CAD build for the part. Positions are in the model's coordinates, mm. A direction names the side the tool comes from. Give positions to 0.01 mm unless a question says otherwise; leave off trailing zeros. Write each loop counter-clockwise with the first axis right and the second up, starting at its lowest first coordinate (ties: lowest second). Pieces come first, ordered by that corner, then holes. Notation, with made-up numbers: (71.5, 32.5) - (114.5, 32.5) arc R10 cw to (114.5, 41.5) - close; hole circle Ø6 at (14, -8). An arc over 180 degrees is marked (long way). Answer as a JSON object with one key per item and string values.
from build123d import *

# Parameters (mm, degrees)
MAIN_CASE_OUTLINE_DEPTH      = 6.02
MAIN_CASE_OUTLINE_DEPTH_BACK = 6.185
SKETCH2_W                    = 78.2
SKETCH2_H                    = 5
GASKET_CUTOUTS_DEPTH         = 4
MAKE_START                   = -9.185
MAKE_ROOM_FOR_BATTERY_DEPTH  = 3
SOLIDIFY_BOTTOM_DEPTH        = 2
MOVE_FACE2_BY                = 15


# Read off the part's stored shape, not the designer's step: Make Room for Battery
with BuildPart() as part:
    # Sketch1 → Main Case Outline (new, two sides: drawn at the far end of the back side and taken through both)
    with BuildSketch(Plane.XY.offset(-MAIN_CASE_OUTLINE_DEPTH_BACK)):
        with BuildLine():
            Line((274.272499626, -45.935), (24.8125, -45.935))
            ThreePointArc((24.8125, -45.935), (20.216304251, -47.838807156), (18.3125, -52.435004109))
            Line((18.3125, -52.435004109), (18.3125, -126.635))
            ThreePointArc((18.3125, -126.635), (20.216307156, -131.231195749), (24.812504109, -133.135))
            Line((24.812504109, -133.135), (274.2725, -133.135))
            ThreePointArc((274.2725, -133.135), (278.868695177, -131.231193416), (280.7725, -126.63499751))
            Line((280.7725, -126.63499751), (280.7725, -52.435))
            ThreePointArc((280.7725, -52.435), (278.868694164, -47.838805571), (274.272499626, -45.935))
        make_face()
        with BuildLine():
            Line((275.7725, -126.635), (275.7725, -52.435))
            ThreePointArc((275.7725, -52.435), (275.333160259, -51.374339477), (274.272499626, -50.935))
            Line((274.272499626, -50.935), (24.8125, -50.935))
            ThreePointArc((24.8125, -50.935), (23.751839477, -51.374339741), (23.3125, -52.435000374))
            Line((23.3125, -52.435000374), (23.3125, -126.635))
            ThreePointArc((23.3125, -126.635), (23.751839741, -127.695660523), (24.812500374, -128.135))
            Line((24.812500374, -128.135), (274.2725, -128.135))
            ThreePointArc((274.2725, -128.135), (275.333160391, -127.695660391), (275.7725, -126.635))
        make_face(mode=Mode.SUBTRACT)
    extrude(amount=MAIN_CASE_OUTLINE_DEPTH + MAIN_CASE_OUTLINE_DEPTH_BACK)

    # Sketch2 → Gasket Cutouts (cut)
    with BuildSketch(Plane.XY.offset(6.02)):
        with Locations((101.9175, -130.635)):
            Rectangle(SKETCH2_W, SKETCH2_H)
        with Locations((216.2175, -130.635)):
            Rectangle(SKETCH2_W, SKETCH2_H)
        with Locations((101.9175, -48.435)):
            Rectangle(SKETCH2_W, SKETCH2_H)
        with Locations((216.2175, -48.435)):
            Rectangle(SKETCH2_W, SKETCH2_H)
    extrude(amount=-GASKET_CUTOUTS_DEPTH, mode=Mode.SUBTRACT)

    # Make Room for Battery outline → Make Room for Battery (add)
    with BuildSketch(Plane.XY.offset(MAKE_START)):
        with BuildLine():
            Line((280.7725, -126.63499751), (280.7725, -52.435))
            ThreePointArc((280.7725, -52.435), (278.868694164, -47.838805571), (274.272499626, -45.935))
            Line((274.272499626, -45.935), (24.8125, -45.935))
            ThreePointArc((24.8125, -45.935), (20.216304251, -47.838807156), (18.3125, -52.435004109))
            Line((18.3125, -52.435004109), (18.3125, -126.635))
            ThreePointArc((18.3125, -126.635), (20.216307156, -131.231195749), (24.812504109, -133.135))
            Line((24.812504109, -133.135), (274.2725, -133.135))
            ThreePointArc((274.2725, -133.135), (278.868695177, -131.231193416), (280.7725, -126.63499751))
        make_face()
        with BuildLine():
            ThreePointArc((275.7725, -126.635), (275.333160391, -127.695660391), (274.2725, -128.135))
            Line((274.2725, -128.135), (24.812500374, -128.135))
            ThreePointArc((24.812500374, -128.135), (23.751839741, -127.695660523), (23.3125, -126.635))
            Line((23.3125, -126.635), (23.3125, -52.435000374))
            ThreePointArc((23.3125, -52.435000374), (23.751839477, -51.374339741), (24.8125, -50.935))
            Line((24.8125, -50.935), (274.272499626, -50.935))
            ThreePointArc((274.272499626, -50.935), (275.333160259, -51.374339477), (275.7725, -52.435))
            Line((275.7725, -52.435), (275.7725, -126.635))
        make_face(mode=Mode.SUBTRACT)
    extrude(amount=MAKE_ROOM_FOR_BATTERY_DEPTH)

    # Sketch3 → Solidify Bottom (add)
    with BuildSketch(Plane(origin=(0, 0, -9.185), x_dir=(-1, 0, 0), z_dir=(0, 0, -1))):
        with BuildLine():
            Line((-280.7725, -52.435), (-280.7725, -126.63499751))
            ThreePointArc((-280.7725, -126.63499751), (-278.868695177, -131.231193416), (-274.2725, -133.135))
            Line((-274.2725, -133.135), (-24.812504109, -133.135))
            ThreePointArc((-24.812504109, -133.135), (-20.216307156, -131.231195749), (-18.3125, -126.635))
            Line((-18.3125, -126.635), (-18.3125, -52.435004109))
            ThreePointArc((-18.3125, -52.435004109), (-20.216304251, -47.838807156), (-24.8125, -45.935))
            Line((-24.8125, -45.935), (-274.272499626, -45.935))
            ThreePointArc((-274.272499626, -45.935), (-278.868694164, -47.838805571), (-280.7725, -52.435))
        make_face()
    extrude(amount=-SOLIDIFY_BOTTOM_DEPTH)

    # Move Face2: a face moved outward by 15.0
    extrude(part.faces().sort_by_distance((149.5425, -89.535, -9.185))[0], amount=MOVE_FACE2_BY, dir=(0, 0, -1))

    # Cut Bottom Face to Angle
    split(bisect_by=Plane(origin=(0, -3.088365547, -25.152718908), x_dir=(-1, 0, 0), z_dir=(2.5491867248569473e-15, -0.12186934340514763, -0.992546151641322)), keep=Keep.BOTTOM)


solid = part.part
Item 1: Probe line 1 (X direction, y = -95, z = 0.75); line 2 (Y direction, x = 31, z = 4) (3 decimals); line 3 (Z direction, x = 78, y = -52) (3 decimals). List the from-to ranges inside material, lowest first. Write a range as from..to.
Entries:
{"line 1": "18.31..23.31, 275.77..280.77", "line 2": "-133.135..-128.135, -50.935..-45.935", "line 3": "-19.147..-7.185"}
Item 2: Flat gauge pins, fed straight in: P1, Ø4.5, axis at y = -47.5, z = 4, coming from the -X side; P2, Ø1.2, axis at y = -48.5, z = 4.5, coming from the +X side; P3, Ø3, axis at y = -131.5, z = 4.5, coming from the -X side; P4, Ø6.5, axis at x = 184, z = 2.5, coming from the +Y side (3 decimals). Where does each tip first touch, or does it go through?
Entries:
{"P1": "x = 18.89", "P2": "x = 279.85", "P3": "x = 19.25", "P4": "y = -45.935"}
Item 3: Cut at C-C (y = -95). Give the cut face in (x, z) (1 decimal), and give its area (3 significant figures).
Entries:
{"outline": "(18.3, -13.9) - (280.8, -13.9) - (280.8, 6) - (275.8, 6) - (275.8, -7.2) - (23.3, -7.2) - (23.3, 6) - (18.3, 6) - close", "area": "1,890 mm2"}
Item 4: Cut at A-A (z = -2.25). Give the cut face in (x, y) (1 decimal), and give its area (3 significant figures).
Entries:
{"outline": "(18.3, -126.6) arc R6.5 ccw to (24.8, -133.1) - (274.3, -133.1) arc R6.5 ccw to (280.8, -126.6) - (280.8, -52.4) arc R6.5 ccw to (274.3, -45.9) - (24.8, -45.9) arc R6.5 ccw to (18.3, -52.4) - close; hole (23.3, -126.6) arc R1.5 ccw to (24.8, -128.1) - (274.3, -128.1) arc R1.5 ccw to (275.8, -126.6) - (275.8, -52.4) arc R1.5 ccw to (274.3, -50.9) - (24.8, -50.9) arc R1.5 ccw to (23.3, -52.4) - close", "area": "3,360 mm2"}
Item 5: Which spindle directions (+Z, -Z, +X, -X, +Y, -Y) get a long thin tool onto all of the face, cutting with end or side? Do faces 1 (the flat face through (151, -89, -7.185)), 2 (the flat face through (148, -133.135, -1)), 3 (the flat face through (101, -48, 2.02)). Say none if no direction does.
Entries:
{"face 1": "+Z", "face 2": "+Z, -Z, +X, -X, -Y", "face 3": "+Z, +Y, -Y"}
Item 6: Cut at D-D (z = -16.25). Give the cut face in (x, y) (1 decimal), and give its area (3 significant figures).
Entries:
{"outline": "(18.3, -75.6) - (280.8, -75.6) - (280.8, -52.4) arc R6.5 ccw to (274.3, -45.9) - (24.8, -45.9) arc R6.5 ccw to (18.3, -52.4) - close", "area": "7,770 mm2"}
Item 7: Mould opens along Y. For faces 4 (the cylindrical face through (20.267, -47.789, -6.755)), 5 (the flat face through (275.772, -89, -1)), 6 (the flat face through (151.38, -88.925, -14.613)) say: +Y half, -Y half, draft (parallel to the pull), parting line (faces both ways), or undercut.
Entries:
{"face 4": "+Y half", "face 5": "undercut", "face 6": "-Y half"}
Item 8: Cut at B-B (x = 146). Give the cut face in (y, z) (3 decimals).
Entries:
{"outline": "(-133.135, -9.185) - (-45.935, -19.892) - (-45.935, 6.02) - (-50.935, 6.02) - (-50.935, -7.185) - (-128.135, -7.185) - (-128.135, 6.02) - (-133.135, 6.02) - close"}
